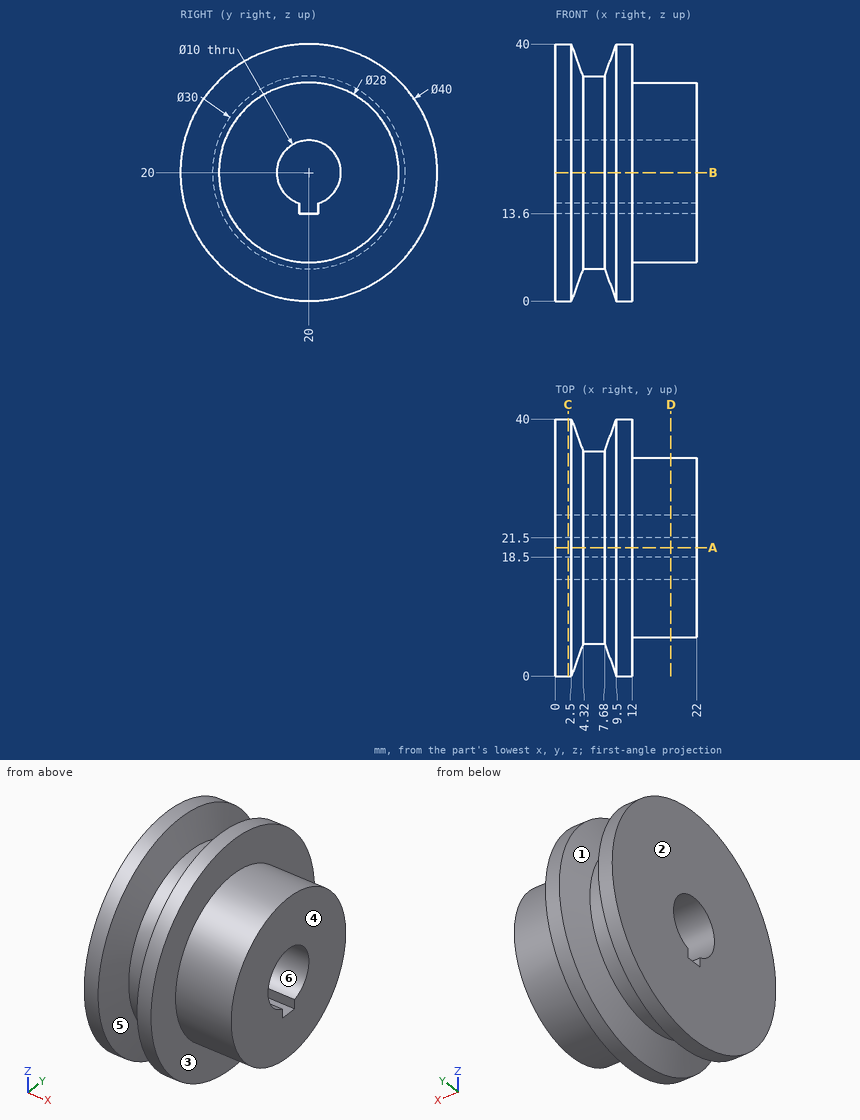
Input: dimensioned drawing with shaded views. Units: mm. Origin: part minimum x, y, z. A direction names the side the tool comes from. Give positions to 0.01 mm unless a question says otherwise; leave off trailing zeros. Order: outer loops, then holes, each group sorted by start corner. A loop starts at its lowest first (then second) coordinate and runs counter-clockwise, first axis right, second up. Notation, with made-up numbers: (44, 58) -> (73, 58) arc R9 ccw to (73, 71) -> close; hole circle Ø2 at (60.5, 37). An arc over 180 degrees is marked (long way). Write item = value, one per line.
Item 1: Mould query, pull axis Z, two halves, no side actions, for the marked faces 4, 5 and 6. Classes: +Z half, -Z half, draft (parallel to the pull), parting line (faces both ways), or undercut.
Check result:
face_4 = draft
face_5 = parting line
face_6 = undercut
Item 2: Section query C-C (x = 2). Output: boundary loops of the cut face in (y, z), then the cut area to 3 significant figures.
Check result:
outline = circle Ø40 at (20, 20); hole (18.5, 13.6) -> (21.5, 13.6) -> (21.5, 15.23) arc R5 ccw (long way) to (18.5, 15.23) -> close
area = 1,170 mm²
Item 3: Section query D-D (x = 18). Output: boundary loops of the cut face in (y, z).
Check result:
outline = circle Ø28 at (20, 20); hole (18.5, 13.6) -> (21.5, 13.6) -> (21.5, 15.23) arc R5 ccw (long way) to (18.5, 15.23) -> close
Item 4: Section query B-B (z = 20). Output: boundary loops of the cut face in (x, y).
Check result:
outline = (0, 0) -> (2.5, 0) -> (4.32, 5) -> (7.68, 5) -> (9.5, 0) -> (12, 0) -> (12, 6) -> (22, 6) -> (22, 15) -> (0, 15) -> close; (0, 25) -> (22, 25) -> (22, 34) -> (12, 34) -> (12, 40) -> (9.5, 40) -> (7.68, 35) -> (4.32, 35) -> (2.5, 40) -> (0, 40) -> close
Item 5: Set-up query: the marked faces 1, 2 and 3. Return all of +Z, -Z, +X, -X, +Y, -Y with unobstructed straight access to the full face (end or side cutting, diameter ignored); none if empty.
Check result:
face_1 = none
face_2 = +Z, -Z, -X, +Y, -Y
face_3 = +X
Item 6: Ray query, probe 1 along Z at (x, y) = (12.25, 20); probe 2 along X at (y, z) = (31, 29); probe 3 along X at (y, z) = (11, 37). Return the intervals inside material, ascending.
Check result:
probe_1 = 6 to 13.6, 25 to 34
probe_2 = 0 to 12
probe_3 = 0 to 2.78, 9.22 to 12
Item 7: Section query A-A (y = 20). Output: boundary loops of the cut face in (x, z).
Check result:
outline = (0, 0) -> (2.5, 0) -> (4.32, 5) -> (7.68, 5) -> (9.5, 0) -> (12, 0) -> (12, 6) -> (22, 6) -> (22, 13.6) -> (0, 13.6) -> close; (0, 25) -> (22, 25) -> (22, 34) -> (12, 34) -> (12, 40) -> (9.5, 40) -> (7.68, 35) -> (4.32, 35) -> (2.5, 40) -> (0, 40) -> close
Item 8: Contact query for flat-ended pins moving along their axis: pin 1 (0.9 mm diameter, centred on x = 10.5, y = 19.5, fed in from +Z); pin 2 (1.8 mm diameter, centred on x = 15, z = 14, fed in from -Y); pin 3 (6 mm diameter, centred on x = 15.5, z = 22.5, fed in from +Y). Output: stop coordinate, or through.
Check result:
pin_1 = 40
pin_2 = 6.96
pin_3 = 34
